Read the model definition and answer for the solid it produces. Units are mm, in the model's axes. A direction names the side the tool comes from. Round coordinates to 2 decimals unless told otherwise and drop trailing zeros. Write each loop counter-clockwise with the first axis right and the second up, starting at its lowest first coordinate (ties: lowest second). Pieces come first, ordered by that corner, then holes. Notation, with made-up numbers: (77.5, 5) - (84.5, 5) arc R22 cw to (84.5, 28) - close; hole circle Ø7 at (-15, 50.25). An arc over 180 degrees is marked (long way). Answer as CSV lines item,"result". Start each with the question number.
1) Find section B-B on z = 0. Determine the outline of the cut face in (x, y), then the cut area to 3 significant figures.
2) Find section D-D on y = 1.25. Determine the outline of the cut face in (x, z).
3) Find section C-C on y = 8. Determine the outline of the cut face in (x, z).
4) For a pull along Z with two mould halves and no side action, classify faces 3 (the flat face through (0, 0, 0)), 4 (the flat face through (0, 1, -11.5)), 5 (the cylindrical face through (2.41, 4.56, -0.57)) as +Z half, -Z half, draft (parallel to the pull), parting line (faces both ways), or undercut.
5) Find section A-A on x = -5. Determine the outline of the cut face in (y, z), then the cut area to 3 significant figures.
6) Which of the six approach directions +Z, -Z, +X, -X, +Y, -Y give full straight-line access (tool end or side, diameter ignored) to faces 1 (the cylindrical face through (-1.63, 5.45, -0.44)), 2 (the flat face through (3, 9, 2))?
7) Consider line 1 along X through (y, z) = (6, 0); line 2 along X through (y, z) = (4.5, -0.75); line 3 along Y through (x, z) = (-9.5, 7.5). Determine where each line is inside the solid, lowest interval first.
from build123d import *

# Parameters (mm, degrees)
BOSS_EXTRUDE1_DEPTH = 2
SKETCH2_R           = 3.4
BOSS_EXTRUDE2_DEPTH = 7
SKETCH3_R           = 2.65
CUT_EXTRUDE1_DEPTH  = 19.587630295


with BuildPart() as part:
    # Sketch1 → Boss-Extrude1 (new body)
    with BuildSketch(Plane(origin=(0, 0, 0), x_dir=(1, 0, 0), z_dir=(0, 1, 0))):
        with BuildLine():
            Line((-9.5, -11.5), (9.5, -11.5))
            ThreePointArc((9.5, -11.5), (10.914213562, -10.914213562), (11.5, -9.5))
            Line((11.5, -9.5), (11.5, 9.5))
            ThreePointArc((11.5, 9.5), (10.914213562, 10.914213562), (9.5, 11.5))
            Line((9.5, 11.5), (-9.5, 11.5))
            ThreePointArc((-9.5, 11.5), (-10.914213562, 10.914213562), (-11.5, 9.5))
            Line((-11.5, 9.5), (-11.5, -9.5))
            ThreePointArc((-11.5, -9.5), (-10.914213562, -10.914213562), (-9.5, -11.5))
        make_face()
    extrude(amount=BOSS_EXTRUDE1_DEPTH)

    # Sketch2 → Boss-Extrude2 (add)
    with BuildSketch(Plane(origin=(0, 2, 0), x_dir=(1, 0, 0), z_dir=(0, 1, 0))):
        with Locations(Location((-5, 0, 0), (0, 0, 270))):
            Circle(SKETCH2_R)
        with Locations(Location((5, 0, 0), (0, 0, 270))):
            Circle(SKETCH2_R)
    extrude(amount=BOSS_EXTRUDE2_DEPTH)

    # Sketch3 → Cut-Extrude1 (cut, through all)
    with BuildSketch(Plane(origin=(0, 9, 0), x_dir=(1, 0, 0), z_dir=(0, 1, 0))):
        with Locations(Location((-5, 0, 0), (0, 0, 270))):
            Circle(SKETCH3_R)
        with Locations(Location((5, 0, 0), (0, 0, 270))):
            Circle(SKETCH3_R)
    extrude(amount=-CUT_EXTRUDE1_DEPTH, mode=Mode.SUBTRACT)


solid = part.part
Check values:
1,outline,"(-11.5, 0) - (-7.65, 0) - (-7.65, 9) - (-8.4, 9) - (-8.4, 2) - (-11.5, 2) - close; (-2.35, 0) - (2.35, 0) - (2.35, 9) - (1.6, 9) - (1.6, 2) - (-1.6, 2) - (-1.6, 9) - (-2.35, 9) - close; (7.65, 0) - (11.5, 0) - (11.5, 2) - (8.4, 2) - (8.4, 9) - (7.65, 9) - close"
1,area,"45.8 mm^2"
2,outline,"(-11.5, -9.5) arc R2 ccw to (-9.5, -11.5) - (9.5, -11.5) arc R2 ccw to (11.5, -9.5) - (11.5, 9.5) arc R2 ccw to (9.5, 11.5) - (-9.5, 11.5) arc R2 ccw to (-11.5, 9.5) - close; hole circle Ø5.3 at (-5, 0); hole circle Ø5.3 at (5, 0)"
3,outline,"circle Ø6.8 at (-5, 0); circle Ø6.8 at (5, 0); hole circle Ø5.3 at (-5, 0); hole circle Ø5.3 at (5, 0)"
4,face 3,"draft"
4,face 4,"-Z half"
4,face 5,"undercut"
5,outline,"(0, -11.5) - (2, -11.5) - (2, -3.4) - (9, -3.4) - (9, -2.65) - (0, -2.65) - close; (0, 2.65) - (9, 2.65) - (9, 3.4) - (2, 3.4) - (2, 11.5) - (0, 11.5) - close"
5,area,"45.9 mm^2"
6,face 1,"+Y"
6,face 2,"+Z, -Z, +X, -X, +Y"
7,line 1,"x = -8.4 to -7.65, -2.35 to -1.6, 1.6 to 2.35, 7.65 to 8.4"
7,line 2,"x = -8.32 to -7.54, -2.46 to -1.68, 1.68 to 2.46, 7.54 to 8.32"
7,line 3,"y = 0 to 2"
